Geometry: final body of the model. Coordinates: model frame, mm. A direction names the side the tool comes from. Give positions to 0.01 mm unless a question says otherwise; leave off trailing zeros. Loops run counter-clockwise (first coordinate to the right, second up) from the corner with the lowest first, then second, coordinate; pieces in that order, holes last. Notation, with made-up numbers: (26.25, 50.25) - (36.25, 50.25) arc R22 cw to (36.25, 59.25) - close; hole circle Ø7 at (19.25, 49.25). An arc over 180 degrees is marked (long way). Use one line per item in the form item = value.
Autodesk Inventor part; units mm, degrees
ref_plane "YZ Plane" through (0, 0, 0) normal (1, 0, 0) x (0, 1, 0)
ref_plane "XZ Plane" through (0, 0, 0) normal (0, 1, 0) x (-1, 0, 0)
ref_plane "XY Plane" through (0, 0, 0) normal (0, 0, 1) x (1, 0, 0)
sketch "Sketch5" plane through (0, 0, 0) normal (0, 1, 0) x (-1, 0, 0)
  line L0 (0, 0) -> (14, 0)
  line L1 (14, 0) -> (14, -14)
  line L2 (14, -14) -> (0, -14)
  line L3 (0, -14) -> (0, 0)
  dimension "d3" = 14
  dimension "d4" = 14
extrude "Extrusion1" add sketch "Sketch5" along normal blind 5
sketch "Sketch6" plane through (0, 5, 0) normal (0, 1, 0) x (1, 0, 0)
  circle A0 centre (-7, 7) radius 5
  line L0 (0, 0) -> (0, 14)
  line L1 (0, 14) -> (-14, 14)
  dimension "d7" = 10
  dimension "d8" = 7
  dimension "d9" = 7
extrude "Extrusion2" add sketch "Sketch6" along normal blind 1
fillet "Fillet1" radius 2 1 edges at (-12, 5, -7)
fillet "Fillet2" radius 1 4 edges at (-14, 2.5, 0) (0, 2.5, 0) (-14, 2.5, -14) (0, 2.5, -14)
fillet "Fillet3" radius 0.5 9 edges at (-12, 6, -7) (-0.2929, 5, -13.7071) (-7, 5, -14) (-13.7071, 5, -13.7071) (-14, 5, -7) (-13.7071, 5, -0.2929) (-7, 5, 0) (-0.2929, 5, -0.2929) (0, 5, -7)
ref_plane "Work Plane2" through (-7, 0, -1) normal (1, 0, 0) x (0, 0, -1)
sketch "Sketch25" plane through (0, 0, 0) normal (0, -1, 0) x (1, 0, 0)
  line L0 (-4, -10) -> (-10, -10)
  line L1 (-10, -10) -> (-10, -4)
  line L2 (-10, -4) -> (-4, -4)
  line L3 (-4, -4) -> (-4, -10)
  line L4 (-1, -14) -> (-13, -14)
  line L5 (0, -1) -> (0, -13)
  point P0 (0, 0)
  dimension "d47" = 6
  dimension "d48" = 6
  dimension "d49" = 4
  dimension "d50" = 4
extrude "Extrusion6" cut sketch "Sketch25" against normal blind 4.5
properties part number "Small_Button"
(1) Cut plane B-B (y = 5.25). Return the cut outline in (x, z).
Solution:
outline = circle Ø11.53 at (-7, -7)
(2) Material intervals for L1, parallel to X at y = 1.75, z = -8.5; L2, parallel to Y at x = -7, z = -6, sorted ascending. Write a range as from..to.
Solution:
L1 = -14..-10, -4..0
L2 = 4.5..6
(3) Pull-direction query (Z, two-part tool) for faces 4 (the face through (-12, 5, -12)), 5 (the face through (-7, 2, -10)), 6 (the face through (-7, 2, -14)); classes: released by +Z, released by -Z, zero draft, split by the parting line, or undercut.
Solution:
face_4 = zero draft
face_5 = undercut
face_6 = released by -Z
(4) Access query for faces 1 (the face through (-10, 2, -7)), 2 (the face through (-2, 5, -12)), 3 (the face through (-2, 5, -2)). Directions: +Z, -Z, +X, -X, +Y, -Y. A direction counts if a zero-diameter tool reaches every point of the face in a straight line with its end or side. Return the directions, or none.
Solution:
face_1 = -Y
face_2 = -Z, +X, +Y
face_3 = +Z, +X, +Y
(5) Pin query (flat end, axial travel): P1, Ø4, axis at x = -12, z = -12, coming from the +Y side. Return the tip coordinate at first contact, or that it passes through.
Solution:
P1 = 5.87
(6) Cut plane A-A (y = 0.5). Return the cut outline in (x, z).
Solution:
outline = (-14, -13) arc R1 ccw to (-13, -14) - (-1, -14) arc R1 ccw to (0, -13) - (0, -1) arc R1 ccw to (-1, 0) - (-13, 0) arc R1 ccw to (-14, -1) - close; hole (-10, -10) - (-4, -10) - (-4, -4) - (-10, -4) - close
